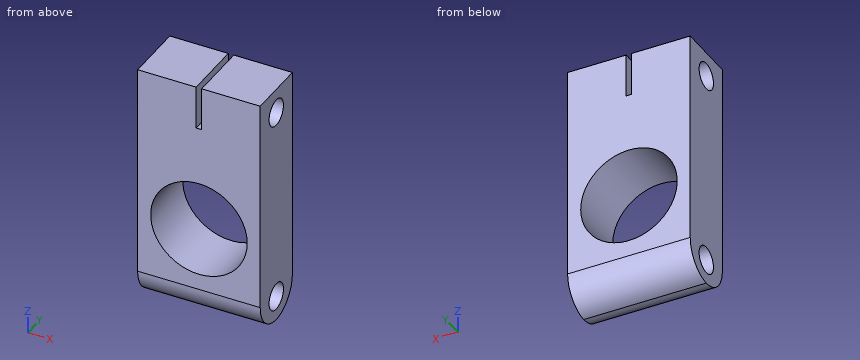
```python
from build123d import *

# Parameters (mm, degrees)
F0_W         = 10.16
F0_H         = 20.32
F2_DEPTH     = 2.5
F1_R         = 4.0005
F3_DEPTH     = 4
F4_R         = 1.1176
F5_DEPTH     = 10.16
F6_W         = 0.4572
F6_H         = 5
F7_DEPTH     = 3.6068
F8_R         = 1.1176
F9_DEPTH     = 10.16
F10_T1_DEPTH = 22.86


# Not quite as in the source:
# - a fillet or chamfer that OpenCascade refuses, or shapes differently, is made with other operations: its cross-section is extruded or revolved along the edge and cut away or added


with BuildPart() as f2:
    # F0 (on Front) → F2 (new body, symmetric)
    with BuildSketch(Plane.XZ):
        Rectangle(F0_W, F0_H)
    extrude(amount=F2_DEPTH, both=True)

    # F1 (on face) → F3 (cut, symmetric)
    with BuildSketch(Plane.XZ):
        with Locations((0, -2.2881471086)):
            Circle(F1_R)
    extrude(amount=F3_DEPTH, both=True, mode=Mode.SUBTRACT)

    # F4 (on face) → F5 (cut)
    with BuildSketch(Plane.YZ.offset(5.08)):
        with Locations((0, -8.1131188199)):
            Circle(F4_R)
    extrude(amount=-F5_DEPTH, mode=Mode.SUBTRACT)

    # F6 (on face) → F7 (cut)
    with BuildSketch(Plane.XY.offset(10.16)):
        Rectangle(F6_W, F6_H)
    extrude(amount=-F7_DEPTH, mode=Mode.SUBTRACT)

    # F8 (on face) → F9 (cut)
    with BuildSketch(Plane.YZ.offset(5.08)):
        with Locations((0, 8.1132977634)):
            Circle(F8_R)
    extrude(amount=-F9_DEPTH, mode=Mode.SUBTRACT)

    # F10: fillet of radius 2.54 on 2 edges, made by hand

    # F10_s2 → F10_t1 (cut)
    with BuildSketch(Plane.YZ.offset(-11.43)):
        with BuildLine():
            ThreePointArc((-0.04, -10.16), (1.7560512242, -9.4160512242), (2.5, -7.62))
            Line((2.5, -7.62), (2.5, -10.16))
            Line((2.5, -10.16), (-0.04, -10.16))
        make_face()
        with BuildLine():
            ThreePointArc((0.04, -10.16), (-1.7560512242, -9.4160512242), (-2.5, -7.62))
            Line((-2.5, -7.62), (-2.5, -10.16))
            Line((-2.5, -10.16), (0.04, -10.16))
        make_face()
    extrude(amount=F10_T1_DEPTH, mode=Mode.SUBTRACT)


solid = f2.part
```
Work out the finished part from the listing and answer in its coordinate system (mm). Coordinates: 2 decimals unless noted, no trailing zeros. Order: outer loops, then holes, each group sorted by start corner. A loop starts at its lowest first (then second) coordinate and runs counter-clockwise, first axis right, second up. Notation, with made-up numbers: M 73.5,-7.75 L 118.5,-7.75 A28 ccw 118.5,12.25 Z; hole C -36,-20.5 d4. An arc over 180 degrees is marked long. Use CSV: the item, a comma, the result in double quotes.
1) Section B-B on z = -5.25 is taken. Write down the section's boundary in (x, y).
Worked out:
outline,"M -5.08,-2.5 L -2.69,-2.5 L -2.69,2.5 L -5.08,2.5 Z; M 2.69,-2.5 L 5.08,-2.5 L 5.08,2.5 L 2.69,2.5 Z"
2) A flat-ended cylindrical pin translates along its axis: pin 1 Ø1 at (x, z) = (0.5, -5.5) entering from +Y. Find the tip coordinate at first contact, or state that the pin passes through.
Worked out:
pin 1,"passes through"
3) Consider line 1 (X direction, y = 0.15, z = -2.25); line 2 (Z direction, x = 0.5, y = 0); line 3 (Z direction, x = -1.2, y = 0). Determine where each line is inside the solid, lowest interval first. Write a range as [from, to].
Worked out:
line 1,"x = [-5.08, -4], [4, 5.08]"
line 2,"z = [-10.16, -9.23], [-7, -6.26], [1.68, 7], [9.23, 10.16]"
line 3,"z = [-10.16, -9.23], [-7, -6.1], [1.53, 7], [9.23, 10.16]"
4) Section C-C on y = -0.45 is taken. Write down the section's boundary in (x, z).
Worked out:
outline,"M -5.08,-10.11 L 5.08,-10.11 L 5.08,-9.14 L -5.08,-9.14 Z; M -5.08,-7.09 L 5.08,-7.09 L 5.08,7.09 L 0.23,7.09 L 0.23,6.55 L -0.23,6.55 L -0.23,7.09 L -5.08,7.09 Z; M -5.08,9.14 L -0.23,9.14 L -0.23,10.16 L -5.08,10.16 Z; M 0.23,9.14 L 5.08,9.14 L 5.08,10.16 L 0.23,10.16 Z; hole C 0,-2.29 d8"
5) Section A-A on x = 2.5 is taken. Write down the section's boundary in (y, z) (3 decimals), plus the area to 3 significant figures.
Worked out:
outline,"M -2.5,-7.62 A2.54 ccw 0,-10.16 A2.54 ccw 2.5,-7.62 L 2.5,-5.411 L -2.5,-5.411 Z; M -2.5,0.835 L 2.5,0.835 L 2.5,10.16 L -2.5,10.16 Z; hole C 0,-8.113 d2.235; hole C 0,8.113 d2.235"
area,"59.8 mm^2"
6) Section D-D on x = 0 is taken. Write down the section's boundary in (y, z), plus the area to 3 significant figures.
Worked out:
outline,"M -2.5,-7.62 A2.54 ccw 0,-10.16 A2.54 ccw 2.5,-7.62 L 2.5,-6.29 L -2.5,-6.29 Z; M -2.5,1.71 L 2.5,1.71 L 2.5,6.55 L -2.5,6.55 Z; hole C 0,-8.11 d2.24"
area,"36.9 mm^2"
